from build123d import *

# Parameters (mm, degrees)
F1_DEPTH             = 22.352
F2_DEPTH             = 79.502
F5_D                 = 19.05
F5_CBORE_D           = 38.1
F5_CBORE_DEPTH       = 3.048
F5_ON_F4_D           = 19.05
F5_ON_F4_CBORE_D     = 38.1
F5_ON_F4_CBORE_DEPTH = 3.048
F6_D                 = 19.05
F6_CSINK_D           = 38.1
F6_CSINK_ANGLE       = 82


with BuildPart() as f1:
    # F0 (on Top) → F1 (new body)
    with BuildSketch(Plane.XY):
        with BuildLine():
            ThreePointArc((25.4, 0), (7.4394877579, 7.4394877579), (0, 25.4))
            Line((0, 25.4), (0, -47.498))
            ThreePointArc((0, -47.498), (7.4394877579, -65.4585122421), (25.4, -72.898))
            Line((25.4, -72.898), (101.6, -72.898))
            ThreePointArc((101.6, -72.898), (119.5605122421, -65.4585122421), (127, -47.498))
            Line((127, -47.498), (127, 25.4))
            ThreePointArc((127, 25.4), (119.5605122421, 7.4394877579), (101.6, 0))
            Line((101.6, 0), (25.4, 0))
        make_face()
    extrude(amount=F1_DEPTH)

    # F0 (on Top) → F2 (join)
    with BuildSketch(Plane.XY):
        with BuildLine():
            Line((0, 143.002), (0, 25.4))
            ThreePointArc((0, 25.4), (7.4394877579, 7.4394877579), (25.4, 0))
            Line((25.4, 0), (101.6, 0))
            ThreePointArc((101.6, 0), (119.5605122421, 7.4394877579), (127, 25.4))
            Line((127, 25.4), (127, 143.002))
            ThreePointArc((127, 143.002), (119.5605122421, 160.9625122421), (101.6, 168.402))
            Line((101.6, 168.402), (25.4, 168.402))
            ThreePointArc((25.4, 168.402), (7.4394877579, 160.9625122421), (0, 143.002))
        make_face()
    extrude(amount=F2_DEPTH)

    # F5 (through all)
    with Locations(Plane.XY.offset(79.502)):
        with Locations((91.948, 127)):
            CounterBoreHole(F5_D / 2, F5_CBORE_D / 2, F5_CBORE_DEPTH)

    # F5 on F4 (through all)
    with Locations(Plane.XY.offset(22.352)):
        with Locations((31.75, -37.846)):
            CounterBoreHole(F5_ON_F4_D / 2, F5_ON_F4_CBORE_D / 2, F5_ON_F4_CBORE_DEPTH)

    # F6 (through all)
    with Locations(Plane.XY.offset(79.502)):
        with Locations((31.75, 79.502), (91.948, 41.402)):
            CounterSinkHole(F6_D / 2, F6_CSINK_D / 2, counter_sink_angle=F6_CSINK_ANGLE)


solid = f1.part
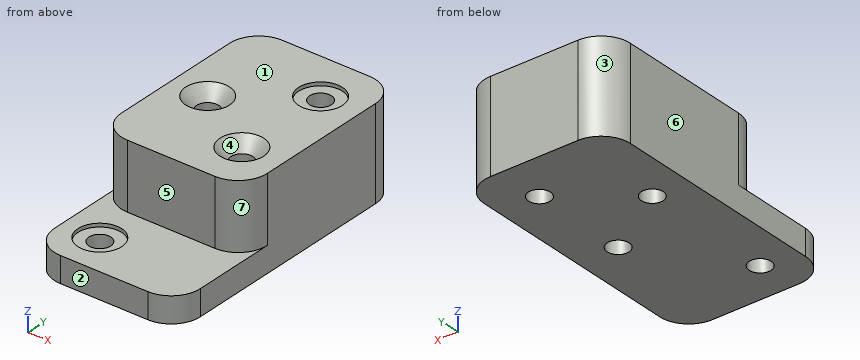
Build history of the part. All positions in model axes, mm. Face numbers are marked on the shaded views. A direction names the side the tool comes from. Round coordinates to 2 decimals unless told otherwise and drop trailing zeros. Write each loop counter-clockwise with the first axis right and the second up, starting at its lowest first coordinate (ties: lowest second). Pieces come first, ordered by that corner, then holes. Notation, with made-up numbers: M -11.75,-18.75 L 38.25,-18.75 A10 cw 38.25,-13.75 Z; hole C 36,69 d7. An arc over 180 degrees is marked long. Answer in a Markdown table with one row per item.
1. Saw through at A-A (x = 31.75). List the corners of the cut face in (y, z), and give its area (3 significant figures).
Geometry check:
| item | result |
|---|---|
| outline | M -72.9,0 L -47.37,0 L -47.37,19.3 L -56.9,19.3 L -56.9,22.35 L -72.9,22.35 Z; M -28.32,0 L 69.98,0 L 69.98,68.54 L 60.45,79.5 L 0,79.5 L 0,22.35 L -18.8,22.35 L -18.8,19.3 L -28.32,19.3 Z; M 89.03,0 L 168.4,0 L 168.4,79.5 L 98.55,79.5 L 89.03,68.54 Z |
| area | 12,900 mm2 |
2. Flat gauge pins, fed straight in: P1, Ø17, axis at x = 91.948, y = 127, coming from the -Z side; P2, Ø5, axis at x = 103, z = 25, coming from the -Y side; P3, Ø8, axis at x = 110, z = 62, coming from the -Y side; P4, Ø4, axis at x = 15, z = 23.5, coming from the +Y side. Where does each tip first touch, or does it go through?
Geometry check:
| item | result |
|---|---|
| P1 | through |
| P2 | y = 0 |
| P3 | y = 0.38 |
| P4 | y = 166.97 |
3. Mould opens along Y. For the marked faces 1, 2, 3 and 4 say: +Y half, -Y half, draft (parallel to the pull), parting line (faces both ways), or undercut.
Geometry check:
| item | result |
|---|---|
| face 1 | draft |
| face 2 | -Y half |
| face 3 | +Y half |
| face 4 | undercut |
4. Probe L1, parallel to Y at x = 91, z = 61.5; L2, parallel to Y at x = 31.75, z = 20.6; L3, parallel to X at y = 35, z = 56. List the from-to ranges inside material, lowest first. Write a range as [from, to].
Geometry check:
| item | result |
|---|---|
| L1 | [0, 31.92], [50.88, 117.52], [136.48, 168.4] |
| L2 | [-72.9, -56.9], [-18.8, 69.98], [89.03, 168.4] |
| L3 | [0, 84.9], [99, 127] |
5. Saw through at B-B (y = 127). List the corners of the cut face in (x, z).
Geometry check:
| item | result |
|---|---|
| outline | M 0,0 L 82.42,0 L 82.42,76.45 L 72.9,76.45 L 72.9,79.5 L 0,79.5 Z; M 101.47,0 L 127,0 L 127,79.5 L 111,79.5 L 111,76.45 L 101.47,76.45 Z |
6. Which spindle directions (+Z, -Z, +X, -X, +Y, -Y) get a long thin tool onto all of the face, cutting with end or side? Do the marked faces 5, 6 and 7. Say none if no direction does.
Geometry check:
| item | result |
|---|---|
| face 5 | +Z, +X, -X, -Y |
| face 6 | +Z, -Z, -X, +Y, -Y |
| face 7 | +Z, +X, -Y |
7. Saw through at C-C (z = 9). List the corners of the cut face in (x, y) (3 decimals).
Geometry check:
| item | result |
|---|---|
| outline | M 0,-47.498 A25.4 ccw 25.4,-72.898 L 101.6,-72.898 A25.4 ccw 127,-47.498 L 127,143.002 A25.4 ccw 101.6,168.402 L 25.4,168.402 A25.4 ccw 0,143.002 Z; hole C 31.75,-37.846 d19.05; hole C 31.75,79.502 d19.05; hole C 91.948,41.402 d19.05; hole C 91.948,127 d19.05 |
8. Saw through at D-D (z = 37). List the corners of the cut face in (x, y) (3 decimals), and give its area (3 significant figures).
Geometry check:
| item | result |
|---|---|
| outline | M 0,25.4 A25.4 ccw 25.4,0 L 101.6,0 A25.4 ccw 127,25.4 L 127,143.002 A25.4 ccw 101.6,168.402 L 25.4,168.402 A25.4 ccw 0,143.002 Z; hole C 31.75,79.502 d19.05; hole C 91.948,41.402 d19.05; hole C 91.948,127 d19.05 |
| area | 20,000 mm2 |
